```python
from build123d import *

# Parameters (mm, degrees)
BOSS_EXTRUDE1_DEPTH     = 10
CUT_EXTRUDE1_DEPTH      = 7
CUT_EXTRUDE3_DEPTH      = 55.838398955
CUT_EXTRUDE3_DEPTH_BACK = 55.838398955
BOSS_EXTRUDE2_DEPTH     = 27
SKETCH6_W               = 13
SKETCH6_H               = 30
CUT_EXTRUDE4_DEPTH      = 107.88879918
FILLET1_R               = 7
FILLET2_R               = 4
SKETCH8_R               = 6.5
CUT_EXTRUDE5_DEPTH      = 27
SKETCH11_R              = 2.15
SKETCH11_W              = 19.8
SKETCH11_H              = 40.5
CUT_EXTRUDE7_DEPTH      = 10
CUT_EXTRUDE8_DEPTH      = 101.056234307
CUT_EXTRUDE8_DEPTH_BACK = 101.056234307
SKETCH12_R              = 10


with BuildPart() as part:
    # Sketch1 → Boss-Extrude1 (new, symmetric)
    with BuildSketch(Plane.XY):
        with BuildLine():
            Line((22.5, 0), (22.5, -49))
            Line((22.5, -49), (-22.5, -49))
            Line((-22.5, -49), (-22.5, 0))
            ThreePointArc((-22.5, 0), (0, 22.5), (22.5, 0))
        make_face()
    extrude(amount=BOSS_EXTRUDE1_DEPTH, both=True)

    # Sketch2 → Cut-Extrude1 (cut)
    with BuildSketch(Plane.XY.offset(10)):
        with BuildLine():
            Line((-19.5, 0), (-17.029582922, -29.598102078))
            ThreePointArc((-17.029582922, -29.598102078), (-1.033858787, -46), (14.96028148, -29.596557582))
            Line((14.96028148, -29.596557582), (19.5, 0))
            ThreePointArc((19.5, 0), (0, 19.5), (-19.5, 0))
        make_face()
    extrude(amount=-CUT_EXTRUDE1_DEPTH, mode=Mode.SUBTRACT)

    # Sketch4 → Cut-Extrude3 (cut, two sides: drawn at the far end of the back side and taken through both)
    with BuildSketch(Plane.ZY.offset(-CUT_EXTRUDE3_DEPTH_BACK)):
        Polygon((10, 0), (10, 22.5), (3, 22.5), align=None)
    extrude(amount=CUT_EXTRUDE3_DEPTH + CUT_EXTRUDE3_DEPTH_BACK, mode=Mode.SUBTRACT)

    # Sketch5 → Boss-Extrude2 (add)
    with BuildSketch(Plane.XY.offset(10)):
        Polygon((-17, -96), (17, -96), (22.5, -49), (-22.5, -49), align=None)
    extrude(amount=-BOSS_EXTRUDE2_DEPTH)

    # Sketch6 → Cut-Extrude4 (cut, through all)
    with BuildSketch(Plane(origin=(-27.852629229, -3.259350229, 0), x_dir=(0, 0, 1), z_dir=(-0.9932225393212899, -0.11622816949504453, 0))):
        with Locations((-3.5, -67.373484893)):
            Rectangle(SKETCH6_W, SKETCH6_H)
    extrude(amount=-CUT_EXTRUDE4_DEPTH, mode=Mode.SUBTRACT)

    # Fillet1
    # the kernel refuses this fillet: 7 mm, written as the material it adds along each edge
    with BuildSketch(Plane(origin=(22.5, -49, -10), x_dir=(0, 1, 0), z_dir=(-1, 0, 0))) as fillet1_piece_1_section:
        with BuildLine():
            CenterArc((FILLET1_R, FILLET1_R), FILLET1_R, 180, 90)
            Line((0, FILLET1_R), (0, 0))
            Line((0, 0), (FILLET1_R, 0))
        make_face()
    fillet1_piece_1 = extrude(amount=45, mode=Mode.PRIVATE)
    fillet1_piece_1 = split(fillet1_piece_1, bisect_by=Plane(origin=(22.378999484, -50.034004412, -11.584712056), z_dir=(-0.9932225393212899, 0.11622816949504457, 0)), keep=Keep.TOP, mode=Mode.PRIVATE)
    fillet1_piece_1 = split(fillet1_piece_1, bisect_by=Plane(origin=(-22.378999484, -50.034004412, -11.584712056), z_dir=(0.9932225393212899, 0.11622816949504457, 0)), keep=Keep.TOP, mode=Mode.PRIVATE)
    add(fillet1_piece_1)

    # Fillet2
    fillet2_edges = [part.edges().sort_by_distance(p)[0] for p in [
        (19.75, -72.5, -17),
        (-19.75, -72.5, -17),
        (-19.75, -72.5, 10),
        (19.75, -72.5, 10),
    ]]
    fillet(fillet2_edges, radius=FILLET2_R)

    # Sketch8 → Cut-Extrude5 (cut)
    with BuildSketch(Plane.XZ.offset(96)):
        with Locations(Location((5.5, -3.5, 0), (0, 0, 270))):
            Circle(SKETCH8_R)
    extrude(amount=-CUT_EXTRUDE5_DEPTH, mode=Mode.SUBTRACT)

    # Sketch11 → Cut-Extrude7 (cut)
    with BuildSketch(Plane.XY.offset(3)):
        with Locations((5.65, 10.804521868)):
            Circle(SKETCH11_R)
        with Locations(Location((-5.65, 10.804521868, 0), (0, 0, 180))):
            Circle(SKETCH11_R)
        with Locations(Location((5.65, -37.595478132, 0), (0, 0, 180))):
            Circle(SKETCH11_R)
        with Locations((-5.65, -37.595478132)):
            Circle(SKETCH11_R)
        with Locations((0, -13.395478132)):
            Rectangle(SKETCH11_W, SKETCH11_H)
    extrude(amount=-CUT_EXTRUDE7_DEPTH, mode=Mode.SUBTRACT)

    # Sketch12 → Cut-Extrude8 (cut, two sides: drawn at the far end of the back side and taken through both)
    with BuildSketch(Plane.XY.offset(-7).offset(-CUT_EXTRUDE8_DEPTH_BACK)):
        with Locations((0, -3.145478132)):
            Circle(SKETCH12_R)
    extrude(amount=CUT_EXTRUDE8_DEPTH + CUT_EXTRUDE8_DEPTH_BACK, mode=Mode.SUBTRACT)


solid = part.part
```
Can you work these out from the model? Positions are in its coordinate system, mm. A direction names the side the tool comes from. Coordinates: 2 decimals unless noted, no trailing zeros. Order: outer loops, then holes, each group sorted by start corner. A loop starts at its lowest first (then second) coordinate and runs counter-clockwise, first axis right, second up.
1. If we section it at A-A (z = -1.25): Please give me the cut outline in (x, y).
2. If we section it at C-C (z = 7.75): Please give me the cut outline in (x, y), then the cut area to 3 significant figures.
3. If we section it at B-B (x = -6): Give the number of separate pieces and of enclosed holes in the cut face, then the cut area to 3 significant figures.
4. I need wall thicknesses on line 1 (Y direction, x = 7, z = -5.5); line 2 (Z direction, x = -8.5, y = -74.5); line 3 (Z direction, x = 3.5, y = 9). Which ranges of each line are inside material? Lowest first, please.
5. For faces 1 (the face through (-6, 11, -7)), 2 (the face through (15, -81.18, -3.59)), 3 (the face through (-18.59, -72.56, -15.8)), which set-ups out of +Z, -Z, +X, -X, +Y, -Y let a thin tool reach every point of the face, with its end or its side?
6. I'm going to push flat-ended pins straight in: pin 1 (6 mm diameter, centred on y = 1.5, z = -6, fed in from -X); pin 2 (4.5 mm diameter, centred on x = 6.5, y = -36.5, fed in from +Z); pin 3 (4 mm diameter, centred on x = -13.5, y = -41, fed in from -Z); pin 4 (2 mm diameter, centred on x = -13, y = -1.5, fed in from -Z). Where does each tip first touch, or does it pass through?
7. Thinking about a two-plate mould opening in Z: for faces 4 (the face through (0, -58, 10)), 5 (the face through (2, -68, 3)), 6 (the face through (-19.177, -77.393, 5.077)), which applies, +Z half, -Z half, draft (parallel to the pull), parting line (faces both ways), or undercut?
Entries:
1. outline: (-22.5, -49) - (-21.77, -55.28) - (22.37, -50.11) - (22.5, -49) - (22.5, 0) arc R22.5 ccw to (-22.5, 0) - close; (-18.28, -85.07) - (-17, -96) - (-0.6, -96) - (-0.6, -83.01) - close; (11.6, -96) - (17, -96) - (18.79, -80.74) - (11.6, -81.58) - close; hole (-9.9, -33.65) - (9.9, -33.65) - (9.9, -4.56) arc R10 ccw to (9.9, -1.73) - (9.9, 6.85) - (-9.9, 6.85) - (-9.9, -1.73) arc R10 ccw to (-9.9, -4.56) - close; hole circle Ø4.3 at (-5.65, -37.6); hole circle Ø4.3 at (-5.65, 10.8); hole circle Ø4.3 at (5.65, -37.6); hole circle Ø4.3 at (5.65, 10.8)
2. outline: (-22.5, -45.53) - (-16.59, -96) - (16.59, -96) - (22.5, -45.53) - (22.5, 0) arc R22.5 ccw to (21.31, 7.23) - (18.11, 7.23) arc R19.5 cw to (19.5, 0) - (14.96, -29.6) arc R16 cw (long way) to (-17.03, -29.6) - (-19.5, 0) arc R19.5 cw to (-18.11, 7.23) - (-21.31, 7.23) arc R22.5 ccw to (-22.5, 0) - close
2. area: 2,600 mm2
3. separate pieces: 2
3. enclosed holes: 1
3. area: 1,300 mm2
4. line 1: y = -51.91 to -39.27, -35.92 to -33.65, 6.85 to 9.13, 12.48 to 21.38
4. line 2: z = -17 to -10, 3 to 10
4. line 3: z = -10 to 3
5. face 1: +Z
5. face 2: -X
5. face 3: -Z, -X, -Y
6. pin 1: stops at x = -22.5
6. pin 2: stops at z = 3
6. pin 3: stops at z = -10.07
6. pin 4: stops at z = -10
7. face 4: +Z half
7. face 5: undercut
7. face 6: draft
